Read the model definition and answer for the solid it produces. Units are mm, in the model's axes. Give positions to 0.01 mm unless a question says otherwise; leave off trailing zeros. Order: outer loops, then holes, each group sorted by start corner. A loop starts at its lowest first (then second) coordinate and runs counter-clockwise, first axis right, second up. Notation, with made-up numbers: (26, 1.25) - (70, 1.25) arc R21 cw to (70, 24.25) - close; hole circle Ø5 at (68, -31.5). An arc over 180 degrees is marked (long way). Return JSON: item names as keys, results as strings.
```python
from build123d import *

# Parameters (mm, degrees)
F0_W     = 50
F0_H     = 10
F1_DEPTH = 300
F2_R     = 4.25
F3_DEPTH = 25
F4_R     = 4
F5_DEPTH = 329


with BuildPart() as f1:
    # F0 (on Right) → F1 (new body)
    with BuildSketch(Plane.YZ):
        Rectangle(F0_W, F0_H)
    extrude(amount=F1_DEPTH)

    # F2 (on face) → F3 (cut)
    with BuildSketch(Plane.XY.offset(5)):
        with Locations((25, 17.5)):
            Circle(F2_R)
        with Locations((275, 17.5)):
            Circle(F2_R)
    extrude(amount=-F3_DEPTH, mode=Mode.SUBTRACT)

    # F4 (on face) → F5 (cut)
    with BuildSketch(Plane.XY.offset(5)):
        with Locations((40, -15)):
            Circle(F4_R)
        with Locations((260, -15)):
            Circle(F4_R)
    extrude(amount=-F5_DEPTH, mode=Mode.SUBTRACT)


solid = f1.part
```
Q1. A cutting plane is placed at A-A (x = 275). Write down the section's boundary in (y, z), and give its area (3 significant figures).
Values:
{"outline": "(-25, -5) - (13.25, -5) - (13.25, 5) - (-25, 5) - close; (21.75, -5) - (25, -5) - (25, 5) - (21.75, 5) - close", "area": "415 mm²"}
Q2. A cutting plane is placed at C-C (x = 40). Write down the section's boundary in (y, z), and give its area (3 significant figures).
Values:
{"outline": "(-25, -5) - (-19, -5) - (-19, 5) - (-25, 5) - close; (-11, -5) - (25, -5) - (25, 5) - (-11, 5) - close", "area": "420 mm²"}
Q3. A cutting plane is placed at D-D (y = 17.5). Write down the section's boundary in (x, z).
Values:
{"outline": "(0, -5) - (20.75, -5) - (20.75, 5) - (0, 5) - close; (29.25, -5) - (270.75, -5) - (270.75, 5) - (29.25, 5) - close; (279.25, -5) - (300, -5) - (300, 5) - (279.25, 5) - close"}
Q4. Consider L1, parallel to X at y = 21, z = 3.5; L2, parallel to X at y = -18.5, z = 1; L3, parallel to Y at x = 275, z = 0.5. Determine where each line is inside the solid, lowest interval first.
Values:
{"L1": "x = 0 to 22.59, 27.41 to 272.59, 277.41 to 300", "L2": "x = 0 to 38.06, 41.94 to 258.06, 261.94 to 300", "L3": "y = -25 to 13.25, 21.75 to 25"}
Q5. A cutting plane is placed at B-B (y = -15). Write down the section's boundary in (x, z).
Values:
{"outline": "(0, -5) - (36, -5) - (36, 5) - (0, 5) - close; (44, -5) - (256, -5) - (256, 5) - (44, 5) - close; (264, -5) - (300, -5) - (300, 5) - (264, 5) - close"}
Q6. Determine the mould class of faces 1 (the cylindrical face through (270.754, 17.687, 0.07)), 2 (the flat face through (148, -25, 0)), 3 (the flat face through (148, 0, 5)) for opening direction Y: released by +Y, released by -Y, zero draft, split by the parting line, or undercut.
Values:
{"face 1": "undercut", "face 2": "released by -Y", "face 3": "zero draft"}
